from build123d import *

# Parameters (mm, degrees)
SKETCH1_R                                      = 22.225
BOSS_EXTRUDE1_DEPTH                            = 5.08
CBORE_FOR_4_SOCKET_HEAD_CAP_SCREW1_D           = 3.2639
CBORE_FOR_4_SOCKET_HEAD_CAP_SCREW1_CBORE_D     = 5.55752
CBORE_FOR_4_SOCKET_HEAD_CAP_SCREW1_CBORE_DEPTH = 2.8448


with BuildPart() as part:
    # Sketch1 → Boss-Extrude1 (new body)
    with BuildSketch(Plane(origin=(0, 0, 0), x_dir=(1, 0, 0), z_dir=(0, 1, 0))):
        with Locations(Location((0, 0, 0), (0, 0, 270))):
            Circle(SKETCH1_R)
    extrude(amount=BOSS_EXTRUDE1_DEPTH)

    # CBORE for #4 Socket Head Cap Screw1 (through all)
    with Locations(Plane(origin=(0, 5.08, 0), x_dir=(1, 0, 0), z_dir=(0, 1, 0))):
        with Locations((-9.525, 0), (-4.7625, 8.248891971), (4.7625, 8.248891971), (9.525, 0), (4.7625, -8.248891971), (-4.7625, -8.248891971)):
            CounterBoreHole(CBORE_FOR_4_SOCKET_HEAD_CAP_SCREW1_D / 2, CBORE_FOR_4_SOCKET_HEAD_CAP_SCREW1_CBORE_D / 2, CBORE_FOR_4_SOCKET_HEAD_CAP_SCREW1_CBORE_DEPTH)


solid = part.part
Geometry: final body of the model. Coordinates: model frame, mm. A direction names the side the tool comes from. Give positions to 0.01 mm unless a question says otherwise; leave off trailing zeros. Order: outer loops, then holes, each group sorted by start corner. A loop starts at its lowest first (then second) coordinate and runs counter-clockwise, first axis right, second up. Notation, with made-up numbers: (33.25, -24) -> (49.25, -24) arc R9 cw to (49.25, -18) -> close; hole circle Ø11 at (15.5, -39). An arc over 180 degrees is marked (long way). Answer as a JSON object with one key per item and string values.
Q1. Material intervals for probe 1 along X at (y, z) = (3.3, 0.5); probe 2 along X at (y, z) = (2.8, 2); probe 3 along Z at (x, y) = (-6.5, 3.65), sorted ascending.
Entries:
{"probe 1": "x = -22.22 to -12.26, -6.79 to 6.79, 12.26 to 22.22", "probe 2": "x = -22.13 to -11.45, -7.6 to 7.6, 11.45 to 22.13", "probe 3": "z = -21.25 to -10.42, -6.08 to 6.08, 10.42 to 21.25"}
Q2. Section B-B (y = 3.15). State how many separate pieces and enclosed holes the cut face has, plus the area to 3 significant figures.
Entries:
{"separate pieces": "1", "enclosed holes": "6", "area": "1,410 mm^2"}
Q3. Access query for faces 4 (the cylindrical face through (-12.3, 3.7, -0.1)), 5 (the flat face through (0, 5.08, 0)). Directions: +Z, -Z, +X, -X, +Y, -Y. A direction counts if a zero-diameter tool reaches every point of the face in a straight line with its end or side. Return the directions, or none.
Entries:
{"face 4": "+Y", "face 5": "+Z, -Z, +X, -X, +Y"}
Q4. Section A-A (z = 0). Output: boundary loops of the cut face in (x, y) (3 decimals), plus the area to 3 significant figures.
Entries:
{"outline": "(-22.225, 0) -> (-11.157, 0) -> (-11.157, 2.235) -> (-12.304, 2.235) -> (-12.304, 5.08) -> (-22.225, 5.08) -> close; (-7.893, 0) -> (7.893, 0) -> (7.893, 2.235) -> (6.746, 2.235) -> (6.746, 5.08) -> (-6.746, 5.08) -> (-6.746, 2.235) -> (-7.893, 2.235) -> close; (11.157, 0) -> (22.225, 0) -> (22.225, 5.08) -> (12.304, 5.08) -> (12.304, 2.235) -> (11.157, 2.235) -> close", "area": "180 mm^2"}
Q5. First-contact query: pin 1 (5 mm diameter, centred on x = 4.76, z = -8.25, fed in from +Y); pin 2 (3 mm diameter, centred on x = -4.76, z = -8.25, fed in from +Y); pin 3 (2 mm diameter, centred on x = 11, y = 1, fed in from +Z). Flat tips, straight axial feed; report the tip coordinate or a pass-through.
Entries:
{"pin 1": "stops at y = 2.24", "pin 2": "passes through", "pin 3": "stops at z = 19.85"}
Q6. Section C-C (x = -16). Output: boundary loops of the cut face in (y, z).
Entries:
{"outline": "(0, -15.43) -> (5.08, -15.43) -> (5.08, 15.43) -> (0, 15.43) -> close"}
Q7. Draft query along Z for faces 1 (the cylindrical face through (18.74, 2.5, 11.95)), 2 (the flat face through (4.7, 2.235, 10.1)), 3 (the flat face through (0, 0, 0)). Return one class per face: released by +Z, released by -Z, zero draft, split by the parting line, or undercut.
Entries:
{"face 1": "split by the parting line", "face 2": "undercut", "face 3": "zero draft"}
Q8. Section D-D (z = 15.5). Output: boundary loops of the cut face in (x, y).
Entries:
{"outline": "(-15.93, 0) -> (15.93, 0) -> (15.93, 5.08) -> (-15.93, 5.08) -> close"}
